```python
from build123d import *

# Parameters (mm, degrees)
F0_W     = 86.9988277555
F0_H     = 59.0435229242
F1_DEPTH = 50.8
F3_W     = 52.5893084705
F3_H     = 35.0492546886
F4_DEPTH = 25.4
F5_W     = 40.0050003082
F5_H     = 26.5801052183
F6_DEPTH = 25.4
F2_R     = 12.0116475693
F7_DEPTH = 25.4
F8_R     = 11.6783182931
F9_DEPTH = 25.4


with BuildPart() as f1:
    # F0 (on Top) → F1 (new body)
    with BuildSketch(Plane.XY):
        Polygon((55.7901114225, 37.7155579627), (-40.3664931655, 37.7155579627), (-40.3664931655, 32.8956767917), (-40.3664931655, -26.1478461325), (-40.3664931655, -32.654684037), (50.9702265263, -32.654684037), (55.7901114225, -32.654684037), (55.7901114225, 32.8956767917), align=None)
        with Locations((7.4708126485, 3.3739153296)):
            Rectangle(F0_W, F0_H, mode=Mode.SUBTRACT)
    extrude(amount=F1_DEPTH)

    # F3 (on face) → F4 (cut)
    with BuildSketch(Plane.XZ.offset(32.654684037)):
        with Locations((8.2922223955, 33.2753726557)):
            Rectangle(F3_W, F3_H)
    extrude(amount=-F4_DEPTH, mode=Mode.SUBTRACT)

    # F5 (on face) → F6 (cut)
    with BuildSketch(Plane(origin=(0, 37.7155579627, 0), x_dir=(-1, 0, 0), z_dir=(0, 1, 0))):
        with Locations((-6.8683279678, 37.5099473909)):
            Rectangle(F5_W, F5_H)
    extrude(amount=-F6_DEPTH, mode=Mode.SUBTRACT)

    # F2 (on face) → F7 (cut)
    with BuildSketch(Plane(origin=(-40.3664931655, 0, 0), x_dir=(0, -1, 0), z_dir=(-1, 0, 0))):
        with Locations((-6.8044061773, 29.7015700489)):
            Circle(F2_R)
    extrude(amount=-F7_DEPTH, mode=Mode.SUBTRACT)

    # F8 (on face) → F9 (cut)
    with BuildSketch(Plane.YZ.offset(55.7901114225)):
        with Locations((3.4555627499, 27.0565394312)):
            Circle(F8_R)
    extrude(amount=-F9_DEPTH, mode=Mode.SUBTRACT)


solid = f1.part
```
Source: CAD feature listing. Evaluate the final solid. Frame: model axes, mm. A direction names the side the tool comes from. Coordinates: 2 decimals unless noted, no trailing zeros. Loops run counter-clockwise (first coordinate to the right, second up) from the corner with the lowest first, then second, coordinate; pieces in that order, holes last. Notation, with made-up numbers: (63.25, 75) -> (68.25, 75) arc R23 ccw to (68.25, 98) -> close; hole circle Ø7 at (23, 32). An arc over 180 degrees is marked (long way). One line per item, written item: value. Start each with the question number.
Q1. Section query A-A, the plane x = 29.5. Return the cut outline in (y, z).
Q2. Section query D-D, the plane z = 13. Return the cut outline in (x, y).
Q3. Contact query for flat-ended pins moving along their axis: P1, Ø7, axis at x = 6, y = -30, coming from the +Z side; P2, Ø21, axis at y = 3.46, z = 27.06, coming from the +X side; P3, Ø4, axis at x = 5, y = 35, coming from the +Z side. Output: stop coordinate, or through.
Q4. Mould query, pull axis Y, two halves, no side actions, for faces 6 (the face through (4, -29, 0)), 7 (the face through (7, -26.148, 14)), 8 (the face through (7, -32.655, 14)). Classes: pulls with the +Y half, pulls with the -Y half, needs draft (parallel to the pull), parting line crosses it, or undercut.
Q5. Line query: line 1 along X through (y, z) = (-25, 7.5); line 2 along Y through (x, z) = (-22, 33.5); line 3 along Y through (x, z) = (34, 45.5). Output: solid intervals per line, ascending.
Q6. Section query C-C, the plane y = 2.5. Return the cut outline in (x, z), and give its area (3 significant figures).
Q7. Section query B-B, the plane z = 40. Return the cut outline in (x, y).
Q8. Set-up query: faces 1 (the face through (-38.23, -4.29, 25.1)), 2 (the face through (7, 35, 24.22)), 3 (the face through (8, -29, 15.751)), 4 (the face through (-36.029, -4, 19)), 5 (the face through (53.414, 0.924, 15.656)). Return all of +Z, -Z, +X, -X, +Y, -Y with unobstructed straight access to the full face (end or side cutting, diameter ignored); none if empty.
Results:
1. outline: (-32.65, 0) -> (-26.15, 0) -> (-26.15, 15.75) -> (-32.65, 15.75) -> close; (32.9, 0) -> (37.72, 0) -> (37.72, 50.8) -> (32.9, 50.8) -> close
2. outline: (-40.37, -32.65) -> (55.79, -32.65) -> (55.79, 37.72) -> (-40.37, 37.72) -> close; hole (-36.03, -26.15) -> (50.97, -26.15) -> (50.97, 32.9) -> (-36.03, 32.9) -> close
3. P1: z = 15.75
3. P2: x = -36.03
3. P3: z = 24.22
4. face 6: needs draft
4. face 7: undercut
4. face 8: pulls with the -Y half
5. line 1: -40.37 to -36.03, 50.97 to 55.79
5. line 2: -32.65 to -26.15, 32.9 to 37.72
5. line 3: 32.9 to 37.72
6. outline: (-40.37, 0) -> (-36.03, 0) -> (-36.03, 18.49) -> (-40.37, 18.49) -> close; (-40.37, 40.92) -> (-36.03, 40.92) -> (-36.03, 50.8) -> (-40.37, 50.8) -> close; (50.97, 0) -> (55.79, 0) -> (55.79, 15.42) -> (50.97, 15.42) -> close; (50.97, 38.7) -> (55.79, 38.7) -> (55.79, 50.8) -> (50.97, 50.8) -> close
6. area: 256 mm^2
7. outline: (-40.37, -32.65) -> (-18, -32.65) -> (-18, -26.15) -> (-36.03, -26.15) -> (-36.03, 0.62) -> (-40.37, 0.62) -> close; (-40.37, 12.99) -> (-36.03, 12.99) -> (-36.03, 32.9) -> (-13.13, 32.9) -> (-13.13, 37.72) -> (-40.37, 37.72) -> close; (26.87, 32.9) -> (50.97, 32.9) -> (50.97, -26.15) -> (34.59, -26.15) -> (34.59, -32.65) -> (55.79, -32.65) -> (55.79, 37.72) -> (26.87, 37.72) -> close
8. face 1: -X
8. face 2: +Z, +Y, -Y
8. face 3: +Z, -Y
8. face 4: +Z, -Z
8. face 5: +X
